from build123d import *

# Parameters (mm, degrees)
BASPROSKE_W        = 12
BASPROSKE_H        = 18
TOOTHCUT_DEPTH     = 29.142494559
TEETHCUTS_COUNT    = 16
TEETHCUTS_ANGLE    = 337.5
BORSKE_R           = 2
BORE_DEPTH         = 50.0000508
SKETCH1_R          = 2
CUT_EXTRUDE1_DEPTH = 18


with BuildPart() as part:
    # BasProSke → Base-Revolve (revolve)
    with BuildSketch(Plane(origin=(0, 0, 0), x_dir=(1, 0, 0), z_dir=(0, 1, 0)), mode=Mode.PRIVATE) as base_revolve_sk:
        with Locations((6, 9)):
            Rectangle(BASPROSKE_W, BASPROSKE_H)
    revolve(base_revolve_sk.sketch.rotate(Axis((-10, 0, 0), (1, 0, 0)), 180), axis=Axis((-10, 0, 0), (1, 0, 0)))

    # TooCutSke → ToothCut (cut, through all)
    with BuildSketch(Plane(origin=(0, 0, 0), x_dir=(0, 0, -1), z_dir=(1, 0, 0))):
        with BuildLine():
            ThreePointArc((1.03434411, 13.459313997), (0, 13.499), (-1.03434411, 13.459313997))
            ThreePointArc((-1.03434411, 13.459313997), (-1.635143665, 15.806872195), (-3.065655864, 17.762792553))
            ThreePointArc((-3.065655864, 17.762792553), (0, 18.0254), (3.065655864, 17.762792553))
            ThreePointArc((3.065655864, 17.762792553), (1.635143665, 15.806872195), (1.03434411, 13.459313997))
        make_face()
    toothcut = extrude(amount=TOOTHCUT_DEPTH, mode=Mode.SUBTRACT)

    # TeethCuts: ToothCut ×16 about axis
    teethcuts_axis = Axis((-10, 0, 0), (1, 0, 0))
    for i in range(1, TEETHCUTS_COUNT):
        add(toothcut.rotate(teethcuts_axis, i * TEETHCUTS_ANGLE / (TEETHCUTS_COUNT - 1)), mode=Mode.SUBTRACT)

    # BorSke → Bore (cut, symmetric)
    with BuildSketch(Plane(origin=(0, 0, 0), x_dir=(0, 0, -1), z_dir=(1, 0, 0))):
        with Locations(Location((0, 0, 0), (0, 0, 180))):
            Circle(BORSKE_R)
    extrude(amount=BORE_DEPTH, both=True, mode=Mode.SUBTRACT)

    # Sketch1 → Cut-Extrude1 (cut)
    with BuildSketch(Plane(origin=(12, 0, 0), x_dir=(0, 0, -1), z_dir=(1, 0, 0))):
        with Locations((0, 8)):
            Circle(SKETCH1_R)
        with Locations((0, -8)):
            Circle(SKETCH1_R)
        with Locations((8, 0)):
            Circle(SKETCH1_R)
        with Locations((-8, 0)):
            Circle(SKETCH1_R)
        with BuildLine():
            Line((2, 1.5), (2, -1.5))
            ThreePointArc((2, -1.5), (-2.5, 0), (2, 1.5))
        make_face()
    extrude(amount=-CUT_EXTRUDE1_DEPTH, mode=Mode.SUBTRACT)


solid = part.part
Could you check a few things on this model? Use its own coordinates, in mm. A direction names the side the tool comes from. Coordinates: 2 decimals unless noted, no trailing zeros. Loops run counter-clockwise (first coordinate to the right, second up) from the corner with the lowest first, then second, coordinate; pieces in that order, holes last.
1. Imagine slicing it at B-B (y = -8). Please give me the cut outline in (x, z), and give its area (3 significant figures).
2. Imagine slicing it at D-D (x = 9.5). Give the number of separate pieces and of enclosed holes in the cut face, and give its area (3 significant figures).
3. For faces 5 (the face through (5.92, 9.56, 9.53)), 6 (the face through (5.92, 1.64, 15.82)), 7 (the face through (5.92, 7.52, -13.94)), which set-ups out of +Z, -Z, +X, -X, +Y, -Y let a thin tool reach every point of the face, with its end or its side?
4. We'd pull the mould along Y, two halves only. Please class faces 1 (the face through (6, 0, -6)), 2 (the face through (12, -4, 0)), 3 (the face through (5.916, -15.762, -1.614)), 4 (the face through (6.084, 3.518, 17.653)): released by +Y, released by -Y, zero draft, split by the parting line, or undercut.
5. Imagine slicing it at A-A (z = 0). Please give me the cut outline in (x, y), and give its area (3 significant figures).
6. For P1, Ø2.5, axis at y = -8, z = 0, coming from the -X side; P2, Ø2, axis at x = 10.5, y = 8.5, coming from the -Z side; P3, Ø5, axis at y = 0, z = -8, coming from the -X side; P4, Ø6, axis at x = 10.5, z = 9, coming from the -Y side, each with a flat end and sliding along its axis, tell me the tip position at first contact or that it passes through.
7. I need wall thicknesses on L1, parallel to Z at x = 3, y = -9.5; L2, parallel to Z at x = 4.75, y = -13; L3, parallel to Z at x = 10.75, y = -14.5. Which ranges of each line are inside material? Lowest first, please.
Computed values:
1. outline: (0, -14.34) - (12, -14.34) - (12, -2) - (0, -2) - close; (0, 2) - (12, 2) - (12, 14.34) - (0, 14.34) - close
1. area: 296 mm2
2. separate pieces: 1
2. enclosed holes: 5
2. area: 700 mm2
3. face 5: +X, -X
3. face 6: +Z, +X, -X
3. face 7: -Z, +X, -X
4. face 1: undercut
4. face 2: zero draft
4. face 3: released by -Y
4. face 4: released by +Y
5. outline: (0, -13.5) - (12, -13.5) - (12, -10) - (0, -10) - close; (0, -6) - (12, -6) - (12, -2.5) - (0, -2.5) - close; (0, 2.5) - (12, 2.5) - (12, 6) - (0, 6) - close; (0, 10) - (12, 10) - (12, 13.5) - (0, 13.5) - close
5. area: 168 mm2
6. P1: passes through
6. P2: stops at z = -15.19
6. P3: stops at x = 0
6. P4: stops at y = -15.23
7. L1: z = -15.19 to -11.23, -9.59 to -1.32, 1.32 to 9.59, 11.23 to 15.19
7. L2: z = -10.22 to -6.68, -4.25 to 4.25, 6.68 to 10.22
7. L3: z = -10.4 to -8.22, -4.53 to -1.18, 1.18 to 4.53, 8.22 to 10.4
